Here's how the part is built. I have some questions about the finished solid (model axes, mm). A direction names the side the tool comes from. Round coordinates to 2 decimals unless told otherwise and drop trailing zeros. Write each loop counter-clockwise with the first axis right and the second up, starting at its lowest first coordinate (ties: lowest second). Pieces come first, ordered by that corner, then holes. Notation, with made-up numbers: (4, 70.25) - (27, 70.25) arc R8 cw to (27, 78.25) - close; hole circle Ø7 at (32, 58.25). An arc over 180 degrees is marked (long way). Return JSON: item names as keys, results as strings. Group by question number.
Autodesk Inventor part; units mm, degrees
ref_plane "YZ Plane" through (0, 0, 0) normal (1, 0, 0) x (0, 1, 0)
ref_plane "XZ Plane" through (0, 0, 0) normal (0, 1, 0) x (-1, 0, 0)
ref_plane "XY Plane" through (0, 0, 0) normal (0, 0, 1) x (1, 0, 0)
sketch "Sketch1" plane through (-446.9925, -258.9913, -45) normal (0, 0, 1) x (1, 0, 0)
  point P0 (521.2387, 184.7451)
sketch "Sketch2" plane through (-446.9925, -258.9913, -45) normal (0, 0, 1) x (1, 0, 0)
  circle A0 centre (446.9925, 258.9913) radius 120
  dimension "d43" = 240
extrude "ExtrusionBlind1" add sketch "Sketch2" along normal blind 90
sketch "Sketch3" plane through (-446.9925, -258.9913, -45) normal (0, 0, 1) x (1, 0, 0)
  circle A0 centre (446.9925, 258.9913) radius 143.9167
  circle A1 centre (446.9925, 258.9913) radius 90
  circle A2 centre (446.9925, 258.9913) radius 120
  dimension "d44" = 287.8334
  dimension "d45" = 180
extrude "ExtrusionBlind2" cut sketch "Sketch3" along normal blind 22 contours A0 | A2
hole "Hole1" at (74.2462, -74.2462, -45) direction (0, 0, 1) diameter 13 end through all
pattern_circular "PolarArray1" count 12 over 360 about axis through (0, 0, -45) along (0, 0, 1) of "Hole1", "Hole1"
sketch "Sketch6" plane through (0, 0, -45) normal (0, 0, -1) x (-1, 0, 0)
  point P0 (0, -30)
sketch "Sketch7" plane through (0, 0, -45) normal (0, 0, -1) x (-1, 0, 0)
  point P0 (-22.5, 5.5)
sketch "Sketch8" plane through (0, 0, 45) normal (0, 0, 1) x (1, 0, 0)
  circle A0 centre (0, 0) radius 80
  circle A1 centre (0, 0) radius 120
  dimension "d42" = 160
extrude "ExtrusionBlind3" cut sketch "Sketch8" against normal blind 45 contours A0
chamfer "Chamfer1" distance 10 angle 45 1 edges at (-90, 0, -45)
hole "Hole2" at (0, -30, -45) direction (0, 0, 1) diameter 10 depth 20 tip angle 118
hole "Hole3" [suppressed]
sketch "Sketch12" plane through (0, 0, -45) normal (0, 0, -1) x (-1, 0, 0)
  line L0 (-2, -119.5) -> (-2, -141.4896)
  line L1 (-2, -141.4896) -> (2, -141.4896)
  line L2 (2, -119.5) -> (2, -141.4896)
  line L3 (2, -119.5) -> (-2, -119.5)
  dimension "d46" = 4
  dimension "d47" = 21.9896
extrude "ExtrusionThru1" cut sketch "Sketch12" against normal through all
properties part number "XL200 PART1" material "Steel, Mild"
1) Imagine slicing it at C-C (z = -29.5). Please give me the cut outline in (x, y).
2) If we mould it in two halves opening along Y, with no side actions, what happens to faces 1 (the cylindrical face through (70.752, 68.765, 11.476)), 2 (the flat face through (-1, 1, -45)), 3 (the cylindrical face through (41.53, 79.845, -29.084))? For each: released by +Y, released by -Y, zero draft, split by the parting line, or undercut.
3) Will these pins go through, and if not, where does the flat tip stop? pin 1 Ø1 at (x, z) = (64, 26.5) entering from -Y; pin 2 Ø4 at (x, y) = (91, -4.5) entering from -Z; pin 3 Ø12 at (x, z) = (63.5, 27.5) entering from +Y.
4) For faces 4 (the cylindrical face through (-32.334, 97.467, 11.476)), 5 (the flat face through (-45, -79, -23)), 6 (the cylindrical face through (-17.34, -78.1, 22.82)), which set-ups out of +Z, -Z, +X, -X, +Y, -Y let a thin tool reach every point of the face, with its end or its side?
5) Imagine slicing it at B-B (x = -101.5). Please give me the cut outline in (y, z).
6) Imagine slicing it at A-A (z = 17). Give the number of separate pieces and of enclosed holes in the cut face, plus the area to 3 significant figures.
7) I need wall thicknesses on line 1 along Y through (x, z) = (29.5, 26.5); line 2 along X through (y, z) = (-106, 24). Which ranges of each line are inside material? Lowest first, please.
Results found:
{
 "1": {"outline": "circle Ø180 at (0, 0); hole circle Ø10 at (0, -30)"},
 "2": {"face 1": "undercut", "face 2": "zero draft", "face 3": "split by the parting line"},
 "3": {"pin 1": "stops at y = -101.82", "pin 2": "stops at z = -35.89", "pin 3": "stops at y = 105.33"},
 "4": {"face 4": "+Z, -Z", "face 5": "-Z", "face 6": "+Z"},
 "5": {"outline": "(-64.01, -23) - (-33.68, -23) - (-33.68, 45) - (-64.01, 45) - close; (-20.68, -23) - (20.68, -23) - (20.68, 45) - (-20.68, 45) - close; (33.68, -23) - (64.01, -23) - (64.01, 45) - (33.68, 45) - close"},
 "6": {"separate pieces": "1", "enclosed holes": "13", "area": "23,500 mm²"},
 "7": {"line 1": "y = -116.32 to -107.49, -95.35 to -74.36, 74.36 to 95.35, 107.49 to 116.32", "line 2": "x = -56.25 to -31.79, -22.56 to 22.56, 31.79 to 56.25"}
}
